```python
from build123d import *

# Parameters (mm, degrees)
SKETCH1_R           = 33
BOSS_EXTRUDE1_DEPTH = 109
SKETCH2_R           = 31
BOSS_EXTRUDE3_DEPTH = 3
BOSS_EXTRUDE4_DEPTH = 3
CUT_EXTRUDE1_START  = -115
SKETCH4_R           = 31
CUT_EXTRUDE1_DEPTH  = 115


with BuildPart() as part:
    # Sketch1 → Boss-Extrude1 (new body)
    with BuildSketch(Plane(origin=(0, 0, 0), x_dir=(1, 0, 0), z_dir=(0, 1, 0))):
        with Locations(Location((0, 0, 0), (0, 0, 270))):
            Circle(SKETCH1_R)
    extrude(amount=BOSS_EXTRUDE1_DEPTH)

    # Sketch2 → Boss-Extrude3 (add)
    with BuildSketch(Plane(origin=(0, 109, 0), x_dir=(1, 0, 0), z_dir=(0, 1, 0))):
        Circle(SKETCH2_R)
        with BuildLine():
            Line((-30.488024573, 12.628553268), (-28.640265508, 11.863186403))
            ThreePointArc((-28.640265508, 11.863186403), (-21.920310217, 21.920310217), (-11.863186403, 28.640265508))
            Line((-11.863186403, 28.640265508), (-12.628553268, 30.488024573))
            ThreePointArc((-12.628553268, 30.488024573), (-23.334523779, 23.334523779), (-30.488024573, 12.628553268))
        make_face()
        with BuildLine():
            ThreePointArc((11.863186403, 28.640265508), (21.920310217, 21.920310217), (28.640265508, 11.863186403))
            Line((28.640265508, 11.863186403), (30.488024573, 12.628553268))
            ThreePointArc((30.488024573, 12.628553268), (23.334523779, 23.334523779), (12.628553268, 30.488024573))
            Line((12.628553268, 30.488024573), (11.863186403, 28.640265508))
        make_face()
        with BuildLine():
            Line((30.488024573, -12.628553268), (28.640265508, -11.863186403))
            ThreePointArc((28.640265508, -11.863186403), (21.920310217, -21.920310217), (11.863186403, -28.640265508))
            Line((11.863186403, -28.640265508), (12.628553268, -30.488024573))
            ThreePointArc((12.628553268, -30.488024573), (23.334523779, -23.334523779), (30.488024573, -12.628553268))
        make_face()
        with BuildLine():
            Line((-12.628553268, -30.488024573), (-11.863186403, -28.640265508))
            ThreePointArc((-11.863186403, -28.640265508), (-21.920310217, -21.920310217), (-28.640265508, -11.863186403))
            Line((-28.640265508, -11.863186403), (-30.488024573, -12.628553268))
            ThreePointArc((-30.488024573, -12.628553268), (-23.334523779, -23.334523779), (-12.628553268, -30.488024573))
        make_face()
    extrude(amount=BOSS_EXTRUDE3_DEPTH)

    # Sketch3 → Boss-Extrude4 (add)
    with BuildSketch(Plane(origin=(0, 112, 0), x_dir=(1, 0, 0), z_dir=(0, 1, 0))):
        with BuildLine():
            Line((-33, 0), (-31, 0))
            ThreePointArc((-31, 0), (-30.404343693, -6.047799982), (-28.640265508, -11.863186403))
            Line((-28.640265508, -11.863186403), (-30.488024573, -12.628553268))
            ThreePointArc((-30.488024573, -12.628553268), (-18.33381769, -27.438497206), (0, -33))
            Line((0, -33), (0, -31))
            ThreePointArc((0, -31), (6.047799982, -30.404343693), (11.863186403, -28.640265508))
            Line((11.863186403, -28.640265508), (12.628553268, -30.488024573))
            ThreePointArc((12.628553268, -30.488024573), (27.438497206, -18.33381769), (33, 0))
            Line((33, 0), (31, 0))
            ThreePointArc((31, 0), (30.404343693, 6.047799982), (28.640265508, 11.863186403))
            Line((28.640265508, 11.863186403), (30.488024573, 12.628553268))
            ThreePointArc((30.488024573, 12.628553268), (18.33381769, 27.438497206), (0, 33))
            Line((0, 33), (0, 31))
            ThreePointArc((0, 31), (-6.047799982, 30.404343693), (-11.863186403, 28.640265508))
            Line((-11.863186403, 28.640265508), (-12.628553268, 30.488024573))
            ThreePointArc((-12.628553268, 30.488024573), (-27.438497206, 18.33381769), (-33, 0))
        make_face()
    extrude(amount=BOSS_EXTRUDE4_DEPTH)

    # Sketch4 → Cut-Extrude1 (cut)
    with BuildSketch(Plane(origin=(0, 115, 0), x_dir=(1, 0, 0), z_dir=(0, 1, 0)).offset(CUT_EXTRUDE1_START)):
        with Locations(Location((0, 0, 0), (0, 0, 270))):
            Circle(SKETCH4_R)
    extrude(amount=CUT_EXTRUDE1_DEPTH, mode=Mode.SUBTRACT)


solid = part.part
```
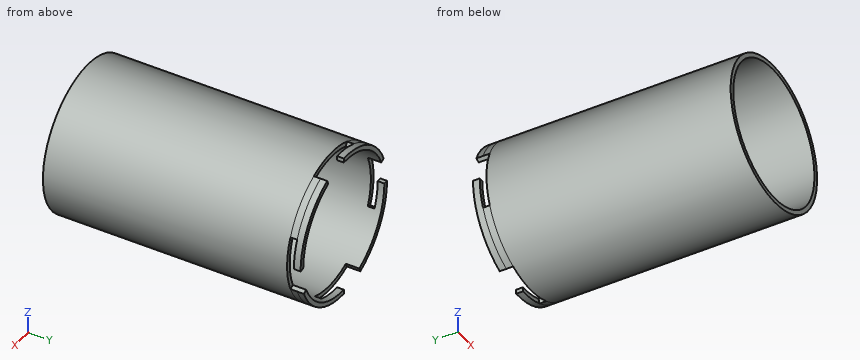
Here's how the part is built. I have some questions about the finished solid (model axes, mm). Coordinates: 2 decimals unless noted, no trailing zeros. Order: outer loops, then holes, each group sorted by start corner. A loop starts at its lowest first (then second) coordinate and runs counter-clockwise, first axis right, second up. Notation, with made-up numbers: M 52,14 L 68,14 A21 cw 68,40 Z; hole C -37,22.5 d11. An arc over 180 degrees is marked long. Answer as a JSON object with one key per item and string values. Group by question number.
(1) Suppose I cut it at D-D, the plane z = -5. Please give me the cut outline in (x, y), then the cut area to 3 significant figures.
(2) I need wall thicknesses on probe 1 along X at (y, z) = (27, 0); probe 2 along Y at (x, z) = (-10, 29.5). Which ranges of each line are inside material? Lowest first, please.
(3) Suppose I cut it at A-A, the plane x = -3.5. Please give me the cut outline in (y, z).
(4) Suppose I cut it at B-B, the plane z = -20. Please give me the cut outline in (x, y).
(5) Suppose I cut it at C-C, the plane y = 50. Please give me the cut outline in (x, z), then the cut area to 3 significant figures.
(6) For pin 1 (0.6 mm diameter, centred on y = 113.5, z = 32, fed in from +X); pin 2 (10 mm diameter, centred on y = 73, z = 11, fed in from +X); pin 3 (12 mm diameter, centred on y = 65.5, z = 24, fed in from -X); pin 4 (5 mm diameter, centred on x = 30.5, z = 8.5, fed in from -Y), each with a flat end and sliding along its axis, tell me the tip position at first contact or that it passes through.
Values found:
{
 "1": {"outline": "M -32.62,0 L -30.59,0 L -30.59,109 L -32.62,109 Z; M -32.62,112 L -30.59,112 L -30.59,115 L -32.62,115 Z; M 30.59,0 L 32.62,0 L 32.62,109 L 30.59,109 Z", "area": "448 mm^2"},
 "2": {"probe 1": "x = -33 to -31, 31 to 33", "probe 2": "y = 0 to 109, 112 to 115"},
 "3": {"outline": "M 0,-32.81 L 109,-32.81 L 109,-30.8 L 0,-30.8 Z; M 0,30.8 L 109,30.8 L 109,32.81 L 0,32.81 Z; M 112,30.8 L 115,30.8 L 115,32.81 L 112,32.81 Z"},
 "4": {"outline": "M -26.25,0 L -23.69,0 L -23.69,115 L -26.25,115 Z; M 23.69,0 L 26.25,0 L 26.25,115 L 23.69,115 Z"},
 "5": {"outline": "C 0,0 d66; hole C 0,0 d62", "area": "402 mm^2"},
 "6": {"pin 1": "stops at x = 0", "pin 2": "stops at x = 32.45", "pin 3": "stops at x = -27.66", "pin 4": "stops at y = 0"}
}
